Here's how the part is built. I have some questions about the finished solid (model axes, mm). Face numbers are marked on the shaded views. A direction names the side the tool comes from. Round coordinates to 2 decimals unless told otherwise and drop trailing zeros. Write each loop counter-clockwise with the first axis right and the second up, starting at its lowest first coordinate (ties: lowest second). Pieces come first, ordered by that corner, then holes. Notation, with made-up numbers: M 19,6 L 40,6 A28 ccw 40,36 Z; hole C 58.5,84 d2. An arc over 180 degrees is marked long. Use a Markdown table: item, result. Add a question column.
```python
from build123d import *

# Parameters (mm, degrees)
SKETCH071_W     = 80
SKETCH071_H     = 84
SKETCH071_R     = 18.5
PAD029_DEPTH    = 6
PAD030_DEPTH    = 80
POCKET027_DEPTH = 84.001
POCKET028_DEPTH = 79.001


with BuildPart() as part:
    # Sketch071 → Pad029 (new body)
    with BuildSketch(Plane.XY):
        Rectangle(SKETCH071_W, SKETCH071_H)
        Circle(SKETCH071_R, mode=Mode.SUBTRACT)
    extrude(amount=PAD029_DEPTH)

    # Sketch072 (on Face3 of Pad029) → Pad030 (join)
    with BuildSketch(Plane(origin=(-40, 0, 0), x_dir=(0, -1, 0), z_dir=(-1, 0, 0))):
        Polygon((27, 0), (42, 0), (42, -15), align=None)
        Polygon((27, 6), (42, 6), (42, 21), align=None)
    extrude(amount=-PAD030_DEPTH)

    # Sketch073 (on Face8 of Pad030) → Pocket027 (cut, through all)
    with BuildSketch(Plane.XZ.offset(42)):
        with BuildLine():
            ThreePointArc((-35.5, 12), (-32.5, 9), (-29.5, 12))
            Line((-29.5, 12), (-29.5, 15))
            ThreePointArc((-29.5, 15), (-32.5, 18), (-35.5, 15))
            Line((-35.5, 12), (-35.5, 15))
        make_face()
        with BuildLine():
            ThreePointArc((35.5, 15), (32.5, 18), (29.5, 15))
            Line((29.5, 15), (29.5, 12))
            ThreePointArc((29.5, 12), (32.5, 9), (35.5, 12))
            Line((35.5, 15), (35.5, 12))
        make_face()
        with BuildLine():
            ThreePointArc((-29.5, -6), (-32.5, -3), (-35.5, -6))
            Line((-35.5, -6), (-35.5, -9))
            ThreePointArc((-35.5, -9), (-32.5, -12), (-29.5, -9))
            Line((-29.5, -6), (-29.5, -9))
        make_face()
        with BuildLine():
            ThreePointArc((35.5, -6), (32.5, -3), (29.5, -6))
            Line((29.5, -6), (29.5, -9))
            ThreePointArc((29.5, -9), (32.5, -12), (35.5, -9))
            Line((35.5, -6), (35.5, -9))
        make_face()
    extrude(amount=-POCKET027_DEPTH, mode=Mode.SUBTRACT)

    # Sketch074 (on Face8 of Pocket027) → Pocket028 (cut, through all)
    with BuildSketch(Plane.XZ.offset(37)):
        with BuildLine():
            ThreePointArc((-27, 15), (-32.5, 20.5), (-38, 15))
            Line((-38, 15), (-38, 12))
            ThreePointArc((-38, 12), (-32.5, 6.5), (-27, 12))
            Line((-27, 15), (-27, 12))
        make_face()
        with BuildLine():
            ThreePointArc((38, 14.79435), (32.5, 20.29435), (27, 14.79435))
            Line((27, 14.79435), (27, 11.79435))
            ThreePointArc((27, 11.79435), (32.5, 6.29435), (38, 11.79435))
            Line((38, 14.79435), (38, 11.79435))
        make_face()
        with BuildLine():
            ThreePointArc((38, -6), (32.5, -0.5), (27, -6))
            Line((27, -6), (27, -9))
            ThreePointArc((27, -9), (32.5, -14.5), (38, -9))
            Line((38, -6), (38, -9))
        make_face()
        with BuildLine():
            ThreePointArc((-27, -6), (-32.5, -0.5), (-38, -6))
            Line((-38, -6), (-38, -9))
            ThreePointArc((-38, -9), (-32.5, -14.5), (-27, -9))
            Line((-27, -6), (-27, -9))
        make_face()
    extrude(amount=-POCKET028_DEPTH, mode=Mode.SUBTRACT)


with BuildPart() as part_1:
    # Body007 placement: moved
    add(part.part.moved(Location((0, -1.2e-05, 103.000008))))


solid = part_1.part
```
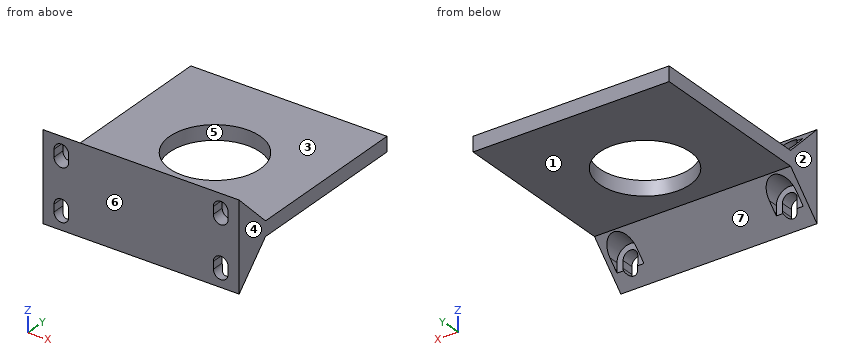
Item 1: I need wall thicknesses on probe 1 along Y at (x, z) = (0, 107.3); probe 2 along X at (y, z) = (-35.5, 102); probe 3 along Y at (x, z) = (-21.5, 118). Which ranges of each line are inside material? Lowest first, please. Write a range as from..to.
Item 2: For pin 1 Ø8 at (x, y) = (7, 31.5) entering from -Z; pin 2 Ø8 at (x, z) = (30, 116.5) entering from +Y; pin 3 Ø1.5 at (x, y) = (-17.5, -22.5) entering from +Z, each with a flat end and sliding along its axis, tell me the tip position at first contact or that it passes through.
Item 3: On a 3-axis mill with a long thin cutter (end or side, diameter ignored), from which of +Z, -Z, +X, -X, +Y, -Y can I reach the whole of each face in a straight line? I mean the marked faces 1, 2 and 3. Say none if no direction works.
Item 4: If we mould it in two halves opening along Y, with no side actions, what happens to the marked faces 4, 5, 6 and 7? For each: +Y half, -Y half, draft (parallel to the pull), parting line (faces both ways), or undercut.
Item 5: Imagine slicing it at D-D on y = -10. List the corners of the cut face in (x, z) for me, plus the area to 3 significant figures.
Item 6: Imagine slicing it at B-B on z = 116.5. List the corners of the cut face in (x, y) for me, plus the area to 3 significant figures.
Item 7: Imagine slicing it at A-A on x = 0. List the corners of the cut face in (y, z) for me.
Item 8: Imagine slicing it at C-C on x = 32.5. List the corners of the cut face in (y, z) for me, plus the area to 3 significant figures.
The answers:
| question | item | result |
|---|---|---|
| 1 | probe 1 | -42..-18.5, 18.5..42 |
| 1 | probe 2 | -40..-34.79, -30.21..30.21, 34.79..40 |
| 1 | probe 3 | -42..-36 |
| 2 | pin 1 | z = 103 |
| 2 | pin 2 | y = -31.74 |
| 2 | pin 3 | z = 109 |
| 3 | face 1 | -Z, +X, -X, +Y |
| 3 | face 2 | +Z, -Z, -X, +Y, -Y |
| 3 | face 3 | +Z, +X, -X, +Y |
| 4 | face 4 | draft |
| 4 | face 5 | undercut |
| 4 | face 6 | -Y half |
| 4 | face 7 | +Y half |
| 5 | outline | M -40,103 L -15.56,103 L -15.56,109 L -40,109 Z; M 15.56,103 L 40,103 L 40,109 L 15.56,109 Z |
| 5 | area | 293 mm² |
| 6 | outline | M -40,-42 L -35.5,-42 L -35.5,-37 L -38,-37 L -38,-34.5 L -40,-34.5 Z; M -29.5,-42 L 29.5,-42 L 29.5,-37 L 27,-37 L 27,-34.5 L -27,-34.5 L -27,-37 L -29.5,-37 Z; M 35.5,-42 L 40,-42 L 40,-34.5 L 38,-34.5 L 38,-37 L 35.5,-37 Z |
| 6 | area | 485 mm² |
| 7 | outline | M -42,88 L -27,103 L -18.5,103 L -18.5,109 L -27,109 L -42,124 Z; M 18.5,103 L 42,103 L 42,109 L 18.5,109 Z |
| 8 | outline | M -42,88 L -39,91 L -42,91 Z; M -42,100 L -37,100 L -37,102.5 L -27.5,102.5 L -27,103 L 42,103 L 42,109 L -27,109 L -27.29,109.29 L -37,109.29 L -37,112 L -42,112 Z; M -42,121 L -39,121 L -42,124 Z |
| 8 | area | 551 mm² |
